Read the model definition and answer for the solid it produces. Units are mm, in the model's axes. A direction names the side the tool comes from. Coordinates: 2 decimals unless noted, no trailing zeros. Write each loop counter-clockwise with the first axis right and the second up, starting at its lowest first coordinate (ties: lowest second). Pieces come first, ordered by that corner, then holes.
from build123d import *

# Parameters (mm, degrees)
SKETCH1_R           = 12.5
BOSS_EXTRUDE1_DEPTH = 44
SKETCH3_R           = 5
CUT_EXTRUDE1_DEPTH  = 10


with BuildPart() as part:
    # Sketch1 → Boss-Extrude1 (new body)
    with BuildSketch(Plane(origin=(0, 0, 0), x_dir=(1, 0, 0), z_dir=(0, 1, 0))):
        Circle(SKETCH1_R)
    extrude(amount=BOSS_EXTRUDE1_DEPTH)

    # Sketch3 → Cut-Extrude1 (cut)
    with BuildSketch(Plane.XZ):
        Circle(SKETCH3_R)
        with BuildLine():
            Line((-5, 11.456439237), (5, 11.456439237))
            ThreePointArc((5, 11.456439237), (0, 12.5), (-5, 11.456439237))
        make_face()
    extrude(amount=-CUT_EXTRUDE1_DEPTH, mode=Mode.SUBTRACT)


solid = part.part
Item 1: The part is cut by section D-D (x = -3.5). Give the vertices of the cut face in (y, z).
Item 2: Determine the mould class of faces 4 (the cylindrical face through (-1.08, 4.93, -4.88)), 5 (the cylindrical face through (-1.627, 21.692, -12.394)), 6 (the flat face through (0, 5, 11.456)) for opening direction X: +X half, -X half, draft (parallel to the pull), parting line (faces both ways), or undercut.
Item 3: For faces 1 (the flat face through (0, 10, 0)), 2 (the flat face through (5.4, 0, -0.7)), 3 (the flat face through (0, 10, 12)), determine the directions among +Z, -Z, +X, -X, +Y, -Y from which every point of the face is accessible in a straight line to the end or side of a thin tool.
Item 4: The part is cut by section C-C (y = 12.5). Give the vertices of the cut face in (x, z).
Item 5: The part is cut by section B-B (x = 0). Give the vertices of the cut face in (y, z), and give its area (3 significant figures).
Item 6: The part is cut by section A-A (z = 0). Give the vertices of the cut face in (x, y), and give its area (3 significant figures).
Item 7: Find the intervals of material crossed by probe 1 along Z at (x, y) = (0, 6.75); probe 2 along Y at (x, z) = (1.25, 4); probe 3 along X at (y, z) = (42, 0.5), in increasing order.
Item 8: Given pin 1 (3 mm diameter, centred on y = 36.5, z = -4.5, fed in from +X); pin 2 (4 mm diameter, centred on y = 9.5, z = -7.5, fed in from +X) (3 decimals); pin 3 (1 mm diameter, centred on x = 9.5, z = 9, fed in from +Y) (3 decimals); pin 4 (1 mm diameter, centred on y = 18.5, z = -6, fed in from -X) (3 decimals), each flat-ended and moving along its own axis, determine where each tip first touches the part or whether it passes through.
Answer:
1. outline: (0, -12) - (44, -12) - (44, 12) - (10, 12) - (10, 11.46) - (0, 11.46) - (0, 3.57) - (10, 3.57) - (10, -3.57) - (0, -3.57) - close
2. face 4: undercut
2. face 5: parting line
2. face 6: draft
3. face 1: -Y
3. face 2: +Z, -Z, +X, -X, -Y
3. face 3: +Z, +X, -X, -Y
4. outline: circle Ø25 at (0, 0)
5. outline: (0, -12.5) - (44, -12.5) - (44, 12.5) - (10, 12.5) - (10, 11.46) - (0, 11.46) - (0, 5) - (10, 5) - (10, -5) - (0, -5) - close
5. area: 990 mm2
6. outline: (-12.5, 0) - (-5, 0) - (-5, 10) - (5, 10) - (5, 0) - (12.5, 0) - (12.5, 44) - (-12.5, 44) - close
6. area: 1,000 mm2
7. probe 1: z = -12.5 to -5, 5 to 11.46
7. probe 2: y = 10 to 44
7. probe 3: x = -12.49 to 12.49
8. pin 1: stops at x = 12.13
8. pin 2: stops at x = 11.225
8. pin 3: passes through
8. pin 4: stops at x = -11.225
